Part model, mm, in its own coordinate system. A direction names the side the tool comes from. Give positions to 0.01 mm unless a question says otherwise; leave off trailing zeros. Write each loop counter-clockwise with the first axis right and the second up, starting at its lowest first coordinate (ties: lowest second). Pieces come first, ordered by that corner, then holes. Notation, with made-up numbers: M 29.5,8.5 L 33.5,8.5 A11 cw 33.5,18.5 Z; hole C 36,72 d7. An arc over 180 degrees is marked long. Use a Markdown table: item, result. Add a question column.
from build123d import *

# Parameters (mm, degrees)
BOSS_EXTRUDE2_DEPTH = 14.5
SKETCH3_R           = 11.1
CUT_EXTRUDE1_DEPTH  = 6
SKETCH5_R           = 4.05
CUT_EXTRUDE2_DEPTH  = 2
SKETCH6_W           = 4.420864072
SKETCH6_H           = 22.2
CUT_EXTRUDE4_DEPTH  = 23.47376248


with BuildPart() as part:
    # Sketch2 → Boss-Extrude2 (new body)
    with BuildSketch(Plane(origin=(0, 0, 0), x_dir=(1, 0, 0), z_dir=(0, 1, 0))):
        with BuildLine():
            Line((-5.794734139, 9.467367969), (-6.679135928, 11.330479613))
            Line((-6.679135928, 11.330479613), (-4.556179387, 12.33822736))
            Line((-4.556179387, 12.33822736), (-3.671777598, 10.475115716))
            ThreePointArc((-3.671777598, 10.475115716), (0, 11.1), (3.671777598, 10.475115716))
            Line((3.671777598, 10.475115716), (4.556179387, 12.33822736))
            Line((4.556179387, 12.33822736), (6.679135928, 11.330479613))
            Line((6.679135928, 11.330479613), (5.794734139, 9.467367969))
            ThreePointArc((5.794734139, 9.467367969), (10.828577002, -2.439655736), (1.175, -11.037634484))
            Line((1.175, -11.037634484), (1.175, -13.1))
            Line((1.175, -13.1), (-1.175, -13.1))
            Line((-1.175, -13.1), (-1.175, -11.037634484))
            ThreePointArc((-1.175, -11.037634484), (-10.828577002, -2.439655736), (-5.794734139, 9.467367969))
        make_face()
    extrude(amount=BOSS_EXTRUDE2_DEPTH)

    # Sketch3 → Cut-Extrude1 (cut)
    with BuildSketch(Plane.XZ):
        Circle(SKETCH3_R)
    extrude(amount=-CUT_EXTRUDE1_DEPTH, mode=Mode.SUBTRACT)

    # Sketch5 → Cut-Extrude2 (cut)
    with BuildSketch(Plane(origin=(0, 14.5, 0), x_dir=(1, 0, 0), z_dir=(0, 1, 0))):
        with Locations(Location((0, 5, 0), (0, 0, 270))):
            Circle(SKETCH5_R)
        with Locations(Location((0, -5, 0), (0, 0, 270))):
            Circle(SKETCH5_R)
    extrude(amount=-CUT_EXTRUDE2_DEPTH, mode=Mode.SUBTRACT)

    # Sketch6 → Cut-Extrude4 (cut, through all)
    with BuildSketch(Plane(origin=(0, 0, 0), x_dir=(1, 0, 0), z_dir=(0, 1, 0))):
        with Locations((8.894567964, 0)):
            Rectangle(SKETCH6_W, SKETCH6_H)
        with Locations((-8.894567964, 0)):
            Rectangle(SKETCH6_W, SKETCH6_H)
    extrude(amount=CUT_EXTRUDE4_DEPTH, mode=Mode.SUBTRACT)


solid = part.part
1. Cut at C-C (z = -5). Write the cut outline in (x, y).
2. Drill centre lines: probe 1 along X at (y, z) = (13.85, -5); probe 2 along Y at (x, z) = (5.25, 6.5); probe 3 along Y at (x, z) = (3.5, -3.75). Where is each one in solid material? Low to high. Write a range as [from, to].
3. Flat gauge pins, fed straight in: pin 1 (0.6 mm diameter, centred on y = 7.5, z = 12, fed in from -X) (3 decimals); pin 2 (5 mm diameter, centred on x = -1, z = 6, fed in from +Y); pin 3 (0.6 mm diameter, centred on y = 4, z = 12.5, fed in from +X) (3 decimals). Where does each tip first touch, or does it go through?
4. Tool access for faces 4 (the flat face through (-6.231, 7.148, -10.386)), 5 (the flat face through (0, 12.5, 5)), 6 (the flat face through (1.175, 7, 12)), 7 (the cylindrical face through (4.745, 2.958, -10.035)): list every direction of +Z, -Z, +X, -X, +Y, -Y with a clear straight run to the whole face (end or side of a thin tool).
5. Cut at B-B (y = 4.75). Write the cut outline in (x, z) (3 decimals).
6. Cut at D-D (x = 0). Write the cut outline in (y, z).
7. Mould opens along Z. For faces 1 (the flat face through (0, 12.5, -5)), 2 (the flat face through (-5.63, 7.15, -11.83)), 3 (the flat face through (-6.684, 10, 0)) say: released by +Z, released by -Z, zero draft, split by the parting line, or undercut.
8. Cut at A-A (y = 13). Write the cut outline in (x, z) (3 decimals), then the cut area to 3 significant figures.
A:
| question | item | result |
|---|---|---|
| 1 | outline | M -6.68,6 L 6.68,6 L 6.68,14.5 L 4.05,14.5 L 4.05,12.5 L -4.05,12.5 L -4.05,14.5 L -6.68,14.5 Z |
| 2 | probe 1 | x = [-6.68, -4.05], [4.05, 6.68] |
| 2 | probe 2 | y = [6, 14.5] |
| 2 | probe 3 | y = [6, 12.5] |
| 3 | pin 1 | stops at x = -1.175 |
| 3 | pin 2 | stops at y = 12.5 |
| 3 | pin 3 | stops at x = 1.175 |
| 4 | face 4 | -X, +Y, -Y |
| 4 | face 5 | +Y |
| 4 | face 6 | +Z, +X, +Y, -Y |
| 4 | face 7 | +Z, -Y |
| 5 | outline | M -6.679,-11.33 L -4.556,-12.338 L -3.672,-10.475 A11.1 cw -5.795,-9.467 Z; M -1.175,11.038 A11.1 cw 1.175,11.038 L 1.175,13.1 L -1.175,13.1 Z; M 3.672,-10.475 L 4.556,-12.338 L 6.679,-11.33 L 5.795,-9.467 A11.1 cw Z |
| 6 | outline | M 0,11.1 L 6,11.1 L 6,-11.1 L 14.5,-11.1 L 14.5,-9.05 L 12.5,-9.05 L 12.5,-0.95 L 14.5,-0.95 L 14.5,0.95 L 12.5,0.95 L 12.5,9.05 L 14.5,9.05 L 14.5,13.1 L 0,13.1 Z |
| 7 | face 1 | undercut |
| 7 | face 2 | released by -Z |
| 7 | face 3 | zero draft |
| 8 | outline | M -6.684,-8.862 A11.1 ccw -5.795,-9.467 L -6.679,-11.33 L -4.556,-12.338 L -3.672,-10.475 A11.1 ccw 3.672,-10.475 L 4.556,-12.338 L 6.679,-11.33 L 5.795,-9.467 A11.1 ccw 6.684,-8.862 L 6.684,8.862 A11.1 ccw 1.175,11.038 L 1.175,13.1 L -1.175,13.1 L -1.175,11.038 A11.1 ccw -6.684,8.862 Z; hole C 0,-5 d8.1; hole C 0,5 d8.1 |
| 8 | area | 189 mm² |
